```python
from build123d import *

# Parameters (mm, degrees)
SKETCH2_R           = 19.05
SKETCH2_R_2         = 12.7
BOSS_EXTRUDE2_DEPTH = 25.4
SKETCH4_W           = 76.2
SKETCH4_H           = 12.7
CUT_EXTRUDE7_DEPTH  = 6.35
CIRPATTERN1_COUNT   = 2
CIRPATTERN1_ANGLE   = 90
SKETCH8_W           = 78.396046772
SKETCH8_H           = 12.7
CUT_EXTRUDE9_DEPTH  = 6.35
CIRPATTERN2_COUNT   = 2
CIRPATTERN2_ANGLE   = 90


with BuildPart() as part:
    # Sketch2 → Boss-Extrude2 (new body)
    with BuildSketch(Plane(origin=(0, 0, 0), x_dir=(1, 0, 0), z_dir=(0, 1, 0))):
        with Locations(Location((0, 0, 0), (0, 0, 270))):
            Circle(SKETCH2_R)
        with Locations(Location((0, 0, 0), (0, 0, 270))):
            Circle(SKETCH2_R_2, mode=Mode.SUBTRACT)
    extrude(amount=BOSS_EXTRUDE2_DEPTH)

    # Sketch4 → Cut-Extrude7 (cut)
    with BuildSketch(Plane(origin=(0, 25.4, 0), x_dir=(1, 0, 0), z_dir=(0, 1, 0))):
        Rectangle(SKETCH4_W, SKETCH4_H)
    cut_extrude7 = extrude(amount=-CUT_EXTRUDE7_DEPTH, mode=Mode.SUBTRACT)

    # CirPattern1: Cut-Extrude7 ×2 about axis
    cirpattern1_axis = Axis((0, 25.4, 0), (0, 1, 0))
    for i in range(1, CIRPATTERN1_COUNT):
        add(cut_extrude7.rotate(cirpattern1_axis, i * CIRPATTERN1_ANGLE / (CIRPATTERN1_COUNT - 1)), mode=Mode.SUBTRACT)

    # Sketch8 → Cut-Extrude9 (cut)
    with BuildSketch(Plane.XZ):
        Rectangle(SKETCH8_W, SKETCH8_H)
    cut_extrude9 = extrude(amount=-CUT_EXTRUDE9_DEPTH, mode=Mode.SUBTRACT)

    # CirPattern2: Cut-Extrude9 ×2 about axis
    cirpattern2_axis = Axis((0, 25.4, 0), (0, -1, 0))
    for i in range(1, CIRPATTERN2_COUNT):
        add(cut_extrude9.rotate(cirpattern2_axis, i * CIRPATTERN2_ANGLE / (CIRPATTERN2_COUNT - 1)), mode=Mode.SUBTRACT)


solid = part.part
```
Geometry: final body of the model. Coordinates: model frame, mm. A direction names the side the tool comes from. Round coordinates to 2 decimals unless told otherwise and drop trailing zeros. Write each loop counter-clockwise with the first axis right and the second up, starting at its lowest first coordinate (ties: lowest second). Pieces come first, ordered by that corner, then holes.
Item 1: Section query D-D (y = 13.5). Return loops of the section in (x, z).
Item 2: Section query C-C (y = 23). Return loops of the section in (x, z), plus the area to 3 significant figures.
Item 3: Set-up query: faces 1 (the face through (-15, 3, 6.35)), 2 (the face through (-6.35, 3, -15)), 3 (the face through (6.35, 22, 15)), 4 (the face through (-15, 22, 6.35)). Return all of +Z, -Z, +X, -X, +Y, -Y with unobstructed straight access to the full face (end or side cutting, diameter ignored); none if empty.
Item 4: Pin query (flat end, axial travel): P1, Ø8, axis at y = 21.5, z = -7, coming from the -X side; P2, Ø7, axis at x = -14.5, y = 2, coming from the -Z side; P3, Ø7, axis at y = 20.5, z = -15.5, coming from the -X side; P4, Ø5, axis at x = -14, z = 8, coming from the -Y side. Return the tip coordinate at first contact, or that it passes through.
Item 5: Mould query, pull axis Z, two halves, no side actions, for faces 5 (the face through (6.35, 3, -15)), 6 (the face through (-15, 3, -6.35)). Classes: +Z half, -Z half, draft (parallel to the pull), parting line (faces both ways), or undercut.
Item 6: Section query A-A (x = 0). Return loops of the section in (y, z), plus the area to 3 significant figures.
Item 7: Section query B-B (z = 0). Return loops of the section in (x, y), plus the area to 3 significant figures.
Item 8: Material intervals for L1, parallel to Z at x = 0, y = 16.75; L2, parallel to Y at x = -2, z = 17, sorted ascending.
Completed:
1. outline: circle Ø38.1 at (0, 0); hole circle Ø25.4 at (0, 0)
2. outline: (-17.96, -6.35) arc R19.05 ccw to (-6.35, -17.96) - (-6.35, -11) arc R12.7 cw to (-11, -6.35) - close; (-17.96, 6.35) - (-11, 6.35) arc R12.7 cw to (-6.35, 11) - (-6.35, 17.96) arc R19.05 ccw to start; (6.35, -17.96) arc R19.05 ccw to (17.96, -6.35) - (11, -6.35) arc R12.7 cw to (6.35, -11) - close; (6.35, 11) arc R12.7 cw to (11, 6.35) - (17.96, 6.35) arc R19.05 ccw to (6.35, 17.96) - close
2. area: 301 mm2
3. face 1: +X, -X, -Y
3. face 2: +Z, -Z, -Y
3. face 3: +Z, -Z, +Y
3. face 4: +X, -X, +Y
4. P1: stops at x = -18.66
4. P2: stops at z = -15.55
4. P3: stops at x = -14.8
4. P4: stops at y = 0
5. face 5: draft
5. face 6: undercut
6. outline: (6.35, -19.05) - (19.05, -19.05) - (19.05, -12.7) - (6.35, -12.7) - close; (6.35, 12.7) - (19.05, 12.7) - (19.05, 19.05) - (6.35, 19.05) - close
6. area: 161 mm2
7. outline: (-19.05, 6.35) - (-12.7, 6.35) - (-12.7, 19.05) - (-19.05, 19.05) - close; (12.7, 6.35) - (19.05, 6.35) - (19.05, 19.05) - (12.7, 19.05) - close
7. area: 161 mm2
8. L1: z = -19.05 to -12.7, 12.7 to 19.05
8. L2: y = 6.35 to 19.05
